Job drawing, mm, ordinate dimensions from the low corner. One solid piece. Coordinates: 2 decimals unless noted, no trailing zeros. Order: outer loops, then holes, each group sorted by start corner. A loop starts at its lowest first (then second) coordinate and runs counter-clockwise, first axis right, second up. Notation, with made-up numbers: (72, 35) - (93, 35) arc R13 ccw to (93, 60) - close; hole circle Ø9 at (17.25, 24). An arc over 180 degrees is marked (long way). Use one line per item in the form item = value.
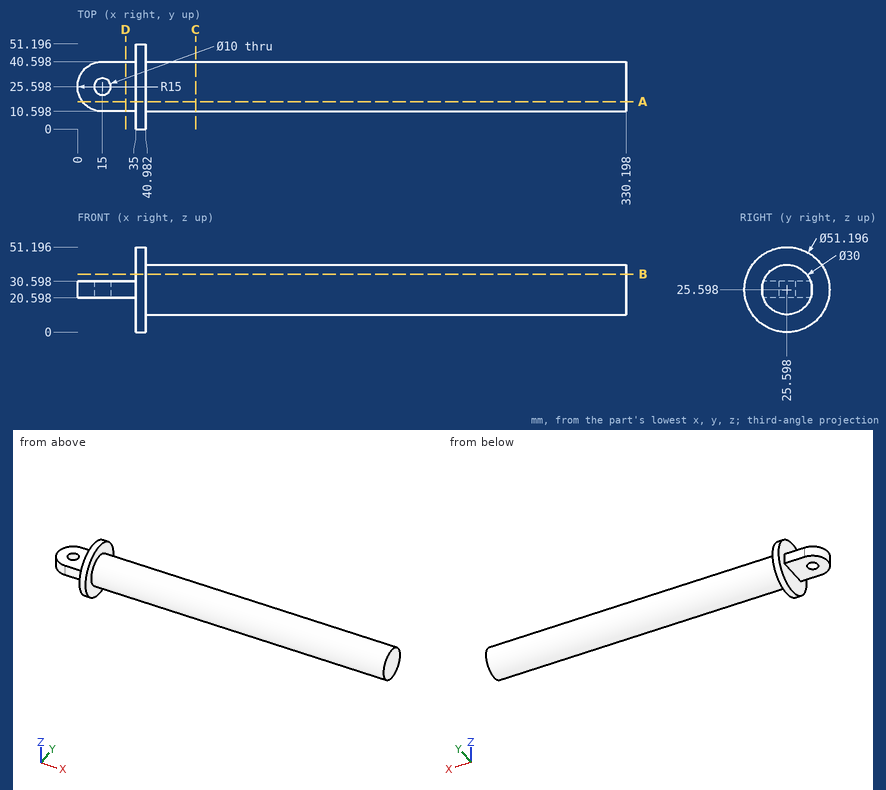
Item 1: Drill centre lines: line 1 (X direction, y = 26, z = 25) (1 decimal); line 2 (Y direction, x = 15, z = 28); line 3 (X direction, y = 28, z = 5.5). Where is each one in solid material? Low to high. Write a range as [from, to].
Derived:
line_1 = [0, 10], [20, 330.2]
line_2 = [10.6, 20.6], [30.6, 40.6]
line_3 = [35, 40.98]
Item 2: Cut at D-D, the plane x = 29. Write the cut outline in (y, z), plus the area to 3 significant figures.
Derived:
outline = (10.6, 20.6) - (40.6, 20.6) - (40.6, 30.6) - (10.6, 30.6) - close
area = 300 mm²
Item 3: Cut at C-C, the plane x = 71. Write the cut outline in (y, z), plus the area to 3 significant figures.
Derived:
outline = circle Ø30 at (25.6, 25.6)
area = 707 mm²
Item 4: Cut at A-A, the plane y = 16.5. Write the cut outline in (x, z) (1 decimal), plus the area to 3 significant figures.
Derived:
outline = (3.1, 20.6) - (35, 20.6) - (35, 1.7) - (41, 1.7) - (41, 13.7) - (330.2, 13.7) - (330.2, 37.5) - (41, 37.5) - (41, 49.5) - (35, 49.5) - (35, 30.6) - (3.1, 30.6) - close
area = 7,500 mm²
Item 5: Drop flat-ended pins along their axis: pin 1 (10 mm diameter, centred on x = 247, z = 23, fed in from +Y); pin 2 (9 mm diameter, centred on x = 21.5, y = 29.5, fed in from +Z); pin 3 (5 mm diameter, centred on x = 199, z = 42, fed in from +Y); pin 4 (4 mm diameter, centred on x = 194.5, y = 7, fed in from -Z). Give the stop position or say it passes through.
Derived:
pin_1 = 40.6
pin_2 = 30.6
pin_3 = 31.23
pin_4 = through
Item 6: Cut at B-B, the plane z = 35. Write the cut outline in (x, y) (1 decimal).
Derived:
outline = (35, 1.8) - (41, 1.8) - (41, 13.9) - (330.2, 13.9) - (330.2, 37.3) - (41, 37.3) - (41, 49.4) - (35, 49.4) - close
